from build123d import *

# Parameters (mm, degrees)
SKETCH_1_R      = 17.5
SKETCH_1_R_2    = 4
SKETCH_1_R_3    = 0.75
EXTRUDE_1_DEPTH = 7.14


with BuildPart() as part:
    # 草图1 → 凸台-拉伸1 (new body)
    with BuildSketch(Plane.XY):
        Circle(SKETCH_1_R)
        Circle(SKETCH_1_R_2, mode=Mode.SUBTRACT)
        with Locations((6.75, 0)):
            Circle(SKETCH_1_R_3, mode=Mode.SUBTRACT)
        with Locations((0, 8.75)):
            Circle(SKETCH_1_R_3, mode=Mode.SUBTRACT)
        with Locations(Location((-6.75, 0, 0), (0, 0, 180))):
            Circle(SKETCH_1_R_3, mode=Mode.SUBTRACT)
        with Locations(Location((0, -8.75, 0), (0, 0, 180))):
            Circle(SKETCH_1_R_3, mode=Mode.SUBTRACT)
    extrude(amount=EXTRUDE_1_DEPTH)


solid = part.part
Here's how the part is built. I have some questions about the finished solid (model axes, mm). Round coordinates to 2 decimals unless told otherwise and drop trailing zeros. Order: outer loops, then holes, each group sorted by start corner. A loop starts at its lowest first (then second) coordinate and runs counter-clockwise, first axis right, second up. Notation, with made-up numbers: M 80,-22.75 L 123,-22.75 A29 cw 123,2.25 Z; hole C 56.5,31 d1. An arc over 180 degrees is marked long. Return JSON: item names as keys, results as strings. Group by question number.
1. If we section it at C-C on z = 1: List the corners of the cut face in (x, y) for me.
2. I'm going to push flat-ended pins straight in: pin 1 Ø3 at (x, z) = (-10.5, 6) entering from +Y; pin 2 Ø1 at (x, z) = (-11.5, 4) entering from +Y; pin 3 Ø1.5 at (x, z) = (-2, 5) entering from +Y. Where does each tip first touch, or does it pass through?
3. If we section it at A-A on x = 0: List the corners of the cut face in (y, z) for me.
4. If we section it at D-D on x = -6.75: List the corners of the cut face in (y, z) for me.
5. If we mould it in two halves opening along X, with no side actions, what happens to faces 1 (the face through (-6, 0, 4)), 2 (the face through (4, -4, 0)), 3 (the face through (-13.887, -10.648, 3.52))? For each: pulls with the +X half, pulls with the -X half, needs draft (parallel to the pull), parting line crosses it, or undercut.
6. If we section it at B-B on y = -3: List the corners of the cut face in (x, z) for me.
7. Please list where these lines run through material, in increasing order: probe 1 along Y at (x, z) = (0, 3.25); probe 2 along X at (y, z) = (2.5, 4.25); probe 3 along Y at (x, z) = (-0.5, 1.5).
Reply:
{
 "1": {"outline": "C 0,0 d35; hole C -6.75,0 d1.5; hole C 0,0 d8; hole C 0,-8.75 d1.5; hole C 0,8.75 d1.5; hole C 6.75,0 d1.5"},
 "2": {"pin 1": "y = 15.01", "pin 2": "y = 13.61", "pin 3": "y = 17.46"},
 "3": {"outline": "M -17.5,0 L -9.5,0 L -9.5,7.14 L -17.5,7.14 Z; M -8,0 L -4,0 L -4,7.14 L -8,7.14 Z; M 4,0 L 8,0 L 8,7.14 L 4,7.14 Z; M 9.5,0 L 17.5,0 L 17.5,7.14 L 9.5,7.14 Z"},
 "4": {"outline": "M -16.15,0 L -0.75,0 L -0.75,7.14 L -16.15,7.14 Z; M 0.75,0 L 16.15,0 L 16.15,7.14 L 0.75,7.14 Z"},
 "5": {"face 1": "undercut", "face 2": "needs draft", "face 3": "parting line crosses it"},
 "6": {"outline": "M -17.24,0 L -2.65,0 L -2.65,7.14 L -17.24,7.14 Z; M 2.65,0 L 17.24,0 L 17.24,7.14 L 2.65,7.14 Z"},
 "7": {"probe 1": "-17.5 to -9.5, -8 to -4, 4 to 8, 9.5 to 17.5", "probe 2": "-17.32 to -3.12, 3.12 to 17.32", "probe 3": "-17.49 to -9.31, -8.19 to -3.97, 3.97 to 8.19, 9.31 to 17.49"}
}
